Could you check a few things on this model? Use its own coordinates, in mm. Round coordinates to 2 decimals unless told otherwise and drop trailing zeros. Write each question's results on one line, items separated by ' | '. Start each with the question number.
1) For P1, Ø3, axis at y = -28, z = 4.5, coming from the +X side; P2, Ø6, axis at x = 0, y = -101.6, coming from the +Z side; P3, Ø1, axis at x = -18, z = 6, coming from the -Y side, each with a flat end and sliding along its axis, tell me the tip position at first contact or that it passes through.
2) Imagine slicing it at A-A, the plane x = 0. Give the number of separate pieces and of enclosed holes in the cut face, plus the area to 3 significant figures.
3) If I drill on probe 1 along Y at (x, z) = (0, 4.25) (1 decimal); probe 2 along Y at (x, z) = (71.5, 1.5); probe 3 along X at (y, z) = (-100, 2.25), over which ranges is the centre line in solid material (lowest first)?
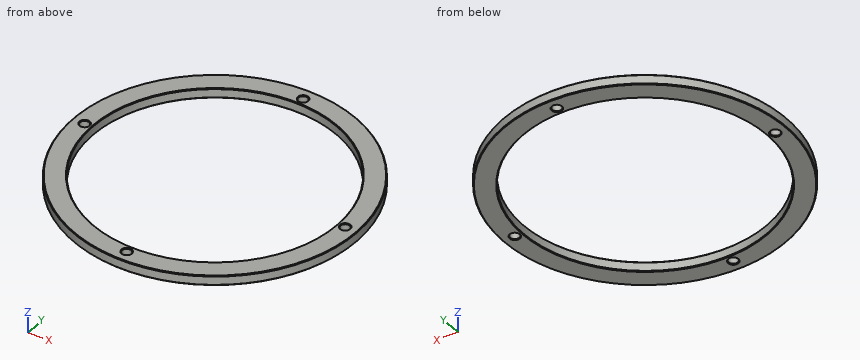
from build123d import *

# Parameters (mm, degrees)
F0_R     = 111.125
F0_R_2   = 95.6945
F1_DEPTH = 7.62
F3_D     = 7.1882
F4_SIZE  = 0.508


with BuildPart() as f1:
    # F0 (on Top) → F1 (new body)
    with BuildSketch(Plane.XY):
        Circle(F0_R)
        Circle(F0_R_2, mode=Mode.SUBTRACT)
    extrude(amount=F1_DEPTH)

    # F3 (through all)
    with Locations(Plane(origin=(0, 0, 0), x_dir=(1, 0, 0), z_dir=(0, 0, -1))):
        with Locations((-101.6, 0), (0, -101.6), (101.6, 0), (0, 101.6)):
            Hole(F3_D / 2)

    # F4
    f4_edges = [f1.edges().sort_by_distance(p)[0] for p in [
        (-111.125, 0, 7.62),
        (-95.6945, 0, 0),
        (-95.6945, 0, 7.62),
        (-111.125, 0, 0),
        (-3.5941, -101.6, 0),
        (-105.1941, 0, 0),
        (98.0059, 0, 0),
        (-3.5941, 101.6, 0),
        (-3.5941, -101.6, 7.62),
        (-105.1941, 0, 7.62),
        (98.0059, 0, 7.62),
        (-3.5941, 101.6, 7.62),
    ]]
    chamfer(f4_edges, length=F4_SIZE)


solid = f1.part
Checked values:
1) P1: x = 107.92 | P2: through | P3: y = -109.74
2) separate pieces: 4 | enclosed holes: 0 | area: 124 mm^2
3) probe 1: -111.1 to -105.2, -98 to -95.7, 95.7 to 98, 105.2 to 111.1 | probe 2: -85.07 to -63.6, 63.6 to 85.07 | probe 3: -48.46 to -3.22, 3.22 to 48.46
